Read the model definition and answer for the solid it produces. Units are mm, in the model's axes. Face numbers are marked on the shaded views. A direction names the side the tool comes from. Round coordinates to 2 decimals unless told otherwise and drop trailing zeros. Write each loop counter-clockwise with the first axis right and the second up, starting at its lowest first coordinate (ties: lowest second). Pieces come first, ordered by that corner, then holes. Notation, with made-up numbers: (3, 64.5) - (43, 64.5) arc R34 ccw to (43, 96.5) - close; hole circle Ø3 at (89, 12.5). An arc over 180 degrees is marked (long way). One line per item, written item: value. Start each with the question number.
(1) Flat-ended cylindrical pins translate along their axes: pin 1 Ø1 at (x, z) = (2, -3) entering from -Y; pin 2 Ø0.9 at (x, z) = (1, -12) entering from -Y. Find the tip coordinate at first contact, or state that the pin passes through.
(2) A cutting plane is placed at C-C, the plane x = 0.9. Determine the outline of the cut face in (y, z), plus the area to 3 significant figures.
(3) A cutting plane is placed at B-B, the plane y = 14. Determine the outline of the cut face in (x, z), plus the area to 3 significant figures.
(4) The mould has two halves that part along Y. Classify the marked faces 4, 5 and 6: +Y half, -Y half, draft (parallel to the pull), parting line (faces both ways), or undercut.
(5) A cutting plane is placed at A-A, the plane z = 1.5. Determine the outline of the cut face in (x, y), plus the area to 3 significant figures.
(6) Find the intervals of material crossed by L1, parallel to Y at x = 1.2, z = -10.5; L2, parallel to Y at x = 2.3, z = 1; L3, parallel to Z at x = 2.3, y = -6.5, in increasing order.
(7) For the marked faces 1, 2 and 3, determine the directions among +Z, -Z, +X, -X, +Y, -Y from which every point of the face is accessible in a straight line to the end or side of a thin tool.
(8) A cutting plane is placed at D-D, the plane y = -16. Determine the outline of the cut face in (x, z).
from build123d import *

# Parameters (mm, degrees)
PAREDEESBOCO_W = 15
PAREDEESBOCO_H = 3
PAREDE_DEPTH   = 3


with BuildPart() as part:
    # ParedeEsboco → Parede (new body)
    with BuildSketch(Plane(origin=(0, 0, 0), x_dir=(0, 0, -1), z_dir=(1, 0, 0))):
        Polygon((13.05, -13.5), (10.05, -13.5), (10.05, -19.5), (4.05, -19.5), (4.05, -16.5), (-4.05, -16.5), (-4.05, -19.5), (-10.05, -19.5), (-10.05, -13.5), (-13.05, -13.5), (-13.05, -7.5), (-10.05, -7.5), (-10.05, -1.5), (-13.05, -1.5), (-13.05, 10.5), (-13.05, 19.5), (13.05, 19.5), (13.05, 10.5), (13.05, -1.5), (10.05, -1.5), (10.05, -7.5), (13.05, -7.5), align=None)
        with Locations((0, 15)):
            Rectangle(PAREDEESBOCO_W, PAREDEESBOCO_H, mode=Mode.SUBTRACT)
    extrude(amount=PAREDE_DEPTH)


solid = part.part
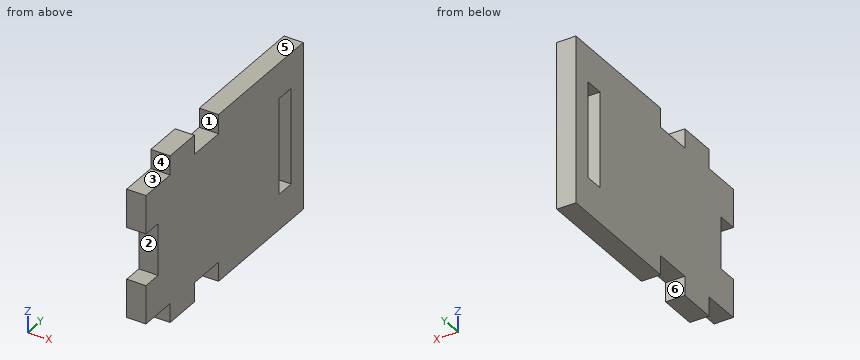
Here are the results:
1. pin 1: y = -16.5
1. pin 2: y = -13.5
2. outline: (-19.5, -10.05) - (-13.5, -10.05) - (-13.5, -13.05) - (-7.5, -13.05) - (-7.5, -10.05) - (-1.5, -10.05) - (-1.5, -13.05) - (19.5, -13.05) - (19.5, 13.05) - (-1.5, 13.05) - (-1.5, 10.05) - (-7.5, 10.05) - (-7.5, 13.05) - (-13.5, 13.05) - (-13.5, 10.05) - (-19.5, 10.05) - (-19.5, 4.05) - (-16.5, 4.05) - (-16.5, -4.05) - (-19.5, -4.05) - close; hole (13.5, -7.5) - (16.5, -7.5) - (16.5, 7.5) - (13.5, 7.5) - close
2. area: 877 mm²
3. outline: (0, -13.05) - (3, -13.05) - (3, -7.5) - (0, -7.5) - close; (0, 7.5) - (3, 7.5) - (3, 13.05) - (0, 13.05) - close
3. area: 33.3 mm²
4. face 4: -Y half
4. face 5: draft
4. face 6: undercut
5. outline: (0, -16.5) - (3, -16.5) - (3, 13.5) - (0, 13.5) - close; (0, 16.5) - (3, 16.5) - (3, 19.5) - (0, 19.5) - close
5. area: 99.0 mm²
6. L1: -13.5 to -7.5, -1.5 to 19.5
6. L2: -16.5 to 13.5, 16.5 to 19.5
6. L3: -10.05 to 10.05
7. face 1: +Z, +X, -X
7. face 2: +X, -X, -Y
7. face 3: +Z, +X, -X, -Y
8. outline: (0, -10.05) - (3, -10.05) - (3, 10.05) - (0, 10.05) - close
